Geometry: final body of the model. Coordinates: model frame, mm. Face numbers are marked on the shaded views. Coordinates: 2 decimals unless noted, no trailing zeros. Order: outer loops, then holes, each group sorted by start corner. A loop starts at its lowest first (then second) coordinate and runs counter-clockwise, first axis right, second up. Notation, with made-up numbers: M 82,72 L 113,72 A22 ccw 113,82 Z; hole C -34,87 d10. An arc over 180 degrees is marked long. One line per question, with ' | ' between items.
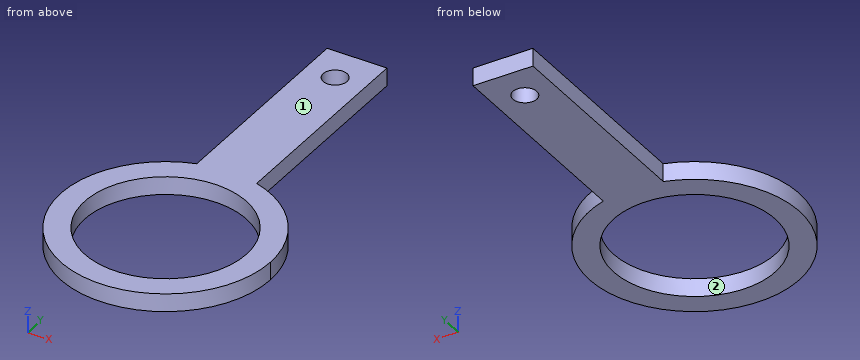
from build123d import *

# Parameters (mm, degrees)
F0_R     = 13.5
F0_R_2   = 2
F1_DEPTH = 3


with BuildPart() as f1:
    # F0 (on Top) → F1 (new body)
    with BuildSketch(Plane.XY):
        with BuildLine():
            ThreePointArc((-5, 16.77051), (-10.45825, -14.031215), (17.5, 0))
            ThreePointArc((17.5, 0), (14.031215, 10.45825), (5, 16.77051))
            ThreePointArc((5, 16.77051), (0, 17.5), (-5, 16.77051))
        make_face()
        Circle(F0_R, mode=Mode.SUBTRACT)
        with BuildLine():
            ThreePointArc((-5, 16.77051), (0, 17.5), (5, 16.77051))
            Line((5, 16.77051), (5, 17.5))
            Line((5, 17.5), (5, 52.5))
            Line((5, 52.5), (-5, 52.5))
            Line((-5, 52.5), (-5, 17.5))
            Line((-5, 17.5), (-5, 16.77051))
        make_face()
        with Locations((0, 46.5)):
            Circle(F0_R_2, mode=Mode.SUBTRACT)
    extrude(amount=F1_DEPTH)


solid = f1.part
1. Draft query along X for the marked faces 1 and 2. Return one class per face: pulls with the +X half, pulls with the -X half, needs draft (parallel to the pull), parting line crosses it, or undercut.
Response values:
face 1: needs draft | face 2: undercut
2. Material intervals for line 1 (Y direction, x = 0, z = 2.25); line 2 (X direction, y = -0.5, z = 1.1); line 3 (Y direction, x = 7.5, z = 1.05), sorted ascending. Write a range as [from, to].
Response values:
line 1: y = [-17.5, -13.5], [13.5, 44.5], [48.5, 52.5] | line 2: x = [-17.49, -13.49], [13.49, 17.49] | line 3: y = [-15.81, -11.22], [11.22, 15.81]
3. Pin query (flat end, axial travel): P1, Ø1, axis at x = -11.5, y = -1.5, coming from the +Z side; P2, Ø0.9, axis at y = 29, z = 1, coming from the -X side. Return the tip coordinate at first contact, or that it passes through.
Response values:
P1: passes through | P2: stops at x = -5
4. Section A-A, the plane z = 0.9. Output: boundary loops of the cut face in (x, y).
Response values:
outline: M -5,16.77 A17.5 ccw long 17.5,0 A17.5 ccw 5,16.77 L 5,52.5 L -5,52.5 Z; hole C 0,0 d27; hole C 0,46.5 d4
5. Section B-B, the plane y = 46.5. Output: boundary loops of the cut face in (x, z), and give its area (3 significant figures).
Response values:
outline: M -5,0 L -2,0 L -2,3 L -5,3 Z; M 2,0 L 5,0 L 5,3 L 2,3 Z | area: 18.0 mm^2
6. Section D-D, the plane x = 0. Output: boundary loops of the cut face in (y, z).
Response values:
outline: M -17.5,0 L -13.5,0 L -13.5,3 L -17.5,3 Z; M 13.5,0 L 44.5,0 L 44.5,3 L 13.5,3 Z; M 48.5,0 L 52.5,0 L 52.5,3 L 48.5,3 Z
7. Section C-C, the plane x = 6.5. Output: boundary loops of the cut face in (y, z), and give its area (3 significant figures).
Response values:
outline: M -16.25,0 L -11.83,0 L -11.83,3 L -16.25,3 Z; M 11.83,0 L 16.25,0 L 16.25,3 L 11.83,3 Z | area: 26.5 mm^2
